from build123d import *

# Parameters (mm, degrees)
SKETCH_1_R      = 3.4
SKETCH_1_R_2    = 3
EXTRUDE_1_DEPTH = 100


with BuildPart() as part:
    # 草图1 → 凸台-拉伸1 (new body)
    with BuildSketch(Plane.XY):
        with BuildLine():
            Line((-5.280003001, 19.242987377), (-15.680003001, 19.242987377))
            ThreePointArc((-15.680003001, 19.242987377), (-18.861983517, 17.924967893), (-20.180003001, 14.742987377))
            Line((-20.180003001, 14.742987377), (-20.180003001, 4.342987377))
            Line((-20.180003001, 4.342987377), (-19.480003001, 4.342987377))
            ThreePointArc((-19.480003001, 4.342987377), (-19.267870967, 4.255119412), (-19.180003001, 4.042987377))
            Line((-19.180003001, 4.042987377), (-19.180003001, 3.342987377))
            Line((-19.180003001, 3.342987377), (-15.980003001, 3.342987377))
            ThreePointArc((-15.980003001, 3.342987377), (-15.767870967, 3.430855343), (-15.680003001, 3.642987377))
            Line((-15.680003001, 3.642987377), (-15.680003001, 6.042987377))
            ThreePointArc((-15.680003001, 6.042987377), (-15.767870967, 6.255119412), (-15.980003001, 6.342987377))
            Line((-15.980003001, 6.342987377), (-16.480003001, 6.342987377))
            ThreePointArc((-16.480003001, 6.342987377), (-17.187109783, 6.635880596), (-17.480003001, 7.342987377))
            Line((-17.480003001, 7.342987377), (-17.480003001, 8.492987377))
            ThreePointArc((-17.480003001, 8.492987377), (-17.187109783, 9.200094158), (-16.480003001, 9.492987377))
            Line((-16.480003001, 9.492987377), (-12.933161007, 9.492987377))
            Line((-12.933161007, 9.492987377), (-8.515789439, 5.07561581))
            ThreePointArc((-8.515789439, 5.07561581), (-8.082243936, 4.426769112), (-7.930003001, 3.661402247))
            Line((-7.930003001, 3.661402247), (-7.930003001, -5.175427493))
            ThreePointArc((-7.930003001, -5.175427493), (-8.082243936, -5.940794357), (-8.515789439, -6.589641055))
            Line((-8.515789439, -6.589641055), (-12.933161007, -11.007012623))
            Line((-12.933161007, -11.007012623), (-16.480003001, -11.007012623))
            ThreePointArc((-16.480003001, -11.007012623), (-17.187109783, -10.714119404), (-17.480003001, -10.007012623))
            Line((-17.480003001, -10.007012623), (-17.480003001, -8.857012623))
            ThreePointArc((-17.480003001, -8.857012623), (-17.187109783, -8.149905842), (-16.480003001, -7.857012623))
            Line((-16.480003001, -7.857012623), (-15.980003001, -7.857012623))
            ThreePointArc((-15.980003001, -7.857012623), (-15.767870967, -7.769144657), (-15.680003001, -7.557012623))
            Line((-15.680003001, -7.557012623), (-15.680003001, -5.157012623))
            ThreePointArc((-15.680003001, -5.157012623), (-15.767870967, -4.944880588), (-15.980003001, -4.857012623))
            Line((-15.980003001, -4.857012623), (-19.180003001, -4.857012623))
            Line((-19.180003001, -4.857012623), (-19.180003001, -5.557012623))
            ThreePointArc((-19.180003001, -5.557012623), (-19.267870967, -5.769144657), (-19.480003001, -5.857012623))
            Line((-19.480003001, -5.857012623), (-20.180003001, -5.857012623))
            Line((-20.180003001, -5.857012623), (-20.180003001, -16.257012623))
            ThreePointArc((-20.180003001, -16.257012623), (-18.861983517, -19.438993138), (-15.680003001, -20.757012623))
            Line((-15.680003001, -20.757012623), (-5.280003001, -20.757012623))
            Line((-5.280003001, -20.757012623), (-5.280003001, -20.057012623))
            ThreePointArc((-5.280003001, -20.057012623), (-5.192135036, -19.844880588), (-4.980003001, -19.757012623))
            Line((-4.980003001, -19.757012623), (-4.280003001, -19.757012623))
            Line((-4.280003001, -19.757012623), (-4.280003001, -16.557012623))
            ThreePointArc((-4.280003001, -16.557012623), (-4.367870967, -16.344880588), (-4.580003001, -16.257012623))
            Line((-4.580003001, -16.257012623), (-6.980003001, -16.257012623))
            ThreePointArc((-6.980003001, -16.257012623), (-7.192135036, -16.344880588), (-7.280003001, -16.557012623))
            Line((-7.280003001, -16.557012623), (-7.280003001, -17.057012623))
            ThreePointArc((-7.280003001, -17.057012623), (-7.57289622, -17.764119404), (-8.280003001, -18.057012623))
            Line((-8.280003001, -18.057012623), (-9.430003001, -18.057012623))
            ThreePointArc((-9.430003001, -18.057012623), (-10.137109783, -17.764119404), (-10.430003001, -17.057012623))
            Line((-10.430003001, -17.057012623), (-10.430003001, -13.510170628))
            Line((-10.430003001, -13.510170628), (-6.012631434, -9.09279906))
            ThreePointArc((-6.012631434, -9.09279906), (-5.363784736, -8.659253558), (-4.598417871, -8.507012623))
            Line((-4.598417871, -8.507012623), (4.238411868, -8.507012623))
            ThreePointArc((4.238411868, -8.507012623), (5.003778733, -8.659253558), (5.652625431, -9.09279906))
            Line((5.652625431, -9.09279906), (10.069996999, -13.510170628))
            Line((10.069996999, -13.510170628), (10.069996999, -17.057012623))
            ThreePointArc((10.069996999, -17.057012623), (9.77710378, -17.764119404), (9.069996999, -18.057012623))
            Line((9.069996999, -18.057012623), (7.919996999, -18.057012623))
            ThreePointArc((7.919996999, -18.057012623), (7.212890217, -17.764119404), (6.919996999, -17.057012623))
            Line((6.919996999, -17.057012623), (6.919996999, -16.557012623))
            ThreePointArc((6.919996999, -16.557012623), (6.832129033, -16.344880588), (6.619996999, -16.257012623))
            Line((6.619996999, -16.257012623), (4.219996999, -16.257012623))
            ThreePointArc((4.219996999, -16.257012623), (4.007864964, -16.344880588), (3.919996999, -16.557012623))
            Line((3.919996999, -16.557012623), (3.919996999, -19.757012623))
            Line((3.919996999, -19.757012623), (4.619996999, -19.757012623))
            ThreePointArc((4.619996999, -19.757012623), (4.832129033, -19.844880588), (4.919996999, -20.057012623))
            Line((4.919996999, -20.057012623), (4.919996999, -20.757012623))
            Line((4.919996999, -20.757012623), (15.319996999, -20.757012623))
            ThreePointArc((15.319996999, -20.757012623), (18.501977514, -19.438993138), (19.819996999, -16.257012623))
            Line((19.819996999, -16.257012623), (19.819996999, -5.857012623))
            Line((19.819996999, -5.857012623), (19.119996999, -5.857012623))
            ThreePointArc((19.119996999, -5.857012623), (18.907864964, -5.769144657), (18.819996999, -5.557012623))
            Line((18.819996999, -5.557012623), (18.819996999, -4.857012623))
            Line((18.819996999, -4.857012623), (15.619996999, -4.857012623))
            ThreePointArc((15.619996999, -4.857012623), (15.407864964, -4.944880588), (15.319996999, -5.157012623))
            Line((15.319996999, -5.157012623), (15.319996999, -7.557012623))
            ThreePointArc((15.319996999, -7.557012623), (15.407864964, -7.769144657), (15.619996999, -7.857012623))
            Line((15.619996999, -7.857012623), (16.119996999, -7.857012623))
            ThreePointArc((16.119996999, -7.857012623), (16.82710378, -8.149905842), (17.119996999, -8.857012623))
            Line((17.119996999, -8.857012623), (17.119996999, -10.007012623))
            ThreePointArc((17.119996999, -10.007012623), (16.82710378, -10.714119404), (16.119996999, -11.007012623))
            Line((16.119996999, -11.007012623), (12.573155004, -11.007012623))
            Line((12.573155004, -11.007012623), (8.155783436, -6.589641055))
            ThreePointArc((8.155783436, -6.589641055), (7.722237934, -5.940794357), (7.569996999, -5.175427493))
            Line((7.569996999, -5.175427493), (7.569996999, 3.661402247))
            ThreePointArc((7.569996999, 3.661402247), (7.722237934, 4.426769112), (8.155783436, 5.07561581))
            Line((8.155783436, 5.07561581), (12.573155004, 9.492987377))
            Line((12.573155004, 9.492987377), (16.119996999, 9.492987377))
            ThreePointArc((16.119996999, 9.492987377), (16.82710378, 9.200094158), (17.119996999, 8.492987377))
            Line((17.119996999, 8.492987377), (17.119996999, 7.342987377))
            ThreePointArc((17.119996999, 7.342987377), (16.82710378, 6.635880596), (16.119996999, 6.342987377))
            Line((16.119996999, 6.342987377), (15.619996999, 6.342987377))
            ThreePointArc((15.619996999, 6.342987377), (15.407864964, 6.255119412), (15.319996999, 6.042987377))
            Line((15.319996999, 6.042987377), (15.319996999, 3.642987377))
            ThreePointArc((15.319996999, 3.642987377), (15.407864964, 3.430855343), (15.619996999, 3.342987377))
            Line((15.619996999, 3.342987377), (18.819996999, 3.342987377))
            Line((18.819996999, 3.342987377), (18.819996999, 4.042987377))
            ThreePointArc((18.819996999, 4.042987377), (18.907864964, 4.255119412), (19.119996999, 4.342987377))
            Line((19.119996999, 4.342987377), (19.819996999, 4.342987377))
            Line((19.819996999, 4.342987377), (19.819996999, 14.742987377))
            ThreePointArc((19.819996999, 14.742987377), (18.501977514, 17.924967893), (15.319996999, 19.242987377))
            Line((15.319996999, 19.242987377), (4.919996999, 19.242987377))
            Line((4.919996999, 19.242987377), (4.919996999, 18.542987377))
            ThreePointArc((4.919996999, 18.542987377), (4.832129033, 18.330855343), (4.619996999, 18.242987377))
            Line((4.619996999, 18.242987377), (3.919996999, 18.242987377))
            Line((3.919996999, 18.242987377), (3.919996999, 15.042987377))
            ThreePointArc((3.919996999, 15.042987377), (4.007864964, 14.830855343), (4.219996999, 14.742987377))
            Line((4.219996999, 14.742987377), (6.619996999, 14.742987377))
            ThreePointArc((6.619996999, 14.742987377), (6.832129033, 14.830855343), (6.919996999, 15.042987377))
            Line((6.919996999, 15.042987377), (6.919996999, 15.542987377))
            ThreePointArc((6.919996999, 15.542987377), (7.212890217, 16.250094158), (7.919996999, 16.542987377))
            Line((7.919996999, 16.542987377), (9.069996999, 16.542987377))
            ThreePointArc((9.069996999, 16.542987377), (9.77710378, 16.250094158), (10.069996999, 15.542987377))
            Line((10.069996999, 15.542987377), (10.069996999, 11.996145383))
            Line((10.069996999, 11.996145383), (5.652625431, 7.578773815))
            ThreePointArc((5.652625431, 7.578773815), (5.003778733, 7.145228312), (4.238411868, 6.992987377))
            Line((4.238411868, 6.992987377), (-4.598417871, 6.992987377))
            ThreePointArc((-4.598417871, 6.992987377), (-5.363784736, 7.145228312), (-6.012631434, 7.578773815))
            Line((-6.012631434, 7.578773815), (-10.430003001, 11.996145383))
            Line((-10.430003001, 11.996145383), (-10.430003001, 15.542987377))
            ThreePointArc((-10.430003001, 15.542987377), (-10.137109783, 16.250094158), (-9.430003001, 16.542987377))
            Line((-9.430003001, 16.542987377), (-8.280003001, 16.542987377))
            ThreePointArc((-8.280003001, 16.542987377), (-7.57289622, 16.250094158), (-7.280003001, 15.542987377))
            Line((-7.280003001, 15.542987377), (-7.280003001, 15.042987377))
            ThreePointArc((-7.280003001, 15.042987377), (-7.192135036, 14.830855343), (-6.980003001, 14.742987377))
            Line((-6.980003001, 14.742987377), (-4.580003001, 14.742987377))
            ThreePointArc((-4.580003001, 14.742987377), (-4.367870967, 14.830855343), (-4.280003001, 15.042987377))
            Line((-4.280003001, 15.042987377), (-4.280003001, 18.242987377))
            Line((-4.280003001, 18.242987377), (-4.980003001, 18.242987377))
            ThreePointArc((-4.980003001, 18.242987377), (-5.192135036, 18.330855343), (-5.280003001, 18.542987377))
            Line((-5.280003001, 18.542987377), (-5.280003001, 19.242987377))
        make_face()
        with Locations((-0.180003001, -0.757012623)):
            Circle(SKETCH_1_R, mode=Mode.SUBTRACT)
        with Locations((-15.305003001, 14.367987377)):
            Circle(SKETCH_1_R_2, mode=Mode.SUBTRACT)
        with Locations((14.944996999, 14.367987377)):
            Circle(SKETCH_1_R_2, mode=Mode.SUBTRACT)
        with Locations((-15.305003001, -15.882012623)):
            Circle(SKETCH_1_R_2, mode=Mode.SUBTRACT)
        with Locations((14.944996999, -15.882012623)):
            Circle(SKETCH_1_R_2, mode=Mode.SUBTRACT)
    extrude(amount=EXTRUDE_1_DEPTH)


solid = part.part
Geometry: final body of the model. Coordinates: model frame, mm. A direction names the side the tool comes from. Coordinates: 2 decimals unless noted, no trailing zeros. Write each loop counter-clockwise with the first axis right and the second up, starting at its lowest first coordinate (ties: lowest second). Pieces come first, ordered by that corner, then holes. Notation, with made-up numbers: (67, 1) - (92, 1) arc R5 ccw to (92, 7) - close; hole circle Ø2 at (-16, 30.5). An arc over 180 degrees is marked (long way). Return JSON: item names as keys, results as strings.
Item 1: Pin query (flat end, axial travel): pin 1 Ø1.6 at (x, z) = (18, 51.5) entering from -Y; pin 2 Ø2.5 at (y, z) = (16.5, 26.5) entering from +X; pin 3 Ø0.6 at (y, z) = (-17, 54) entering from -X; pin 4 Ø1 at (x, y) = (14.5, -9.5) entering from +Z. Return the tip coordinate at first contact, or that it passes through.
Completed:
{"pin 1": "stops at y = -20.35", "pin 2": "stops at x = 19.79", "pin 3": "stops at x = -20.16", "pin 4": "passes through"}
Item 2: Section query C-C (z = 36). Count the separate pieces of the cut face and the enclosed holes in it, and give its area (3 significant figures).
Completed:
{"separate pieces": "1", "enclosed holes": "5", "area": "701 mm2"}
Item 3: Section query A-A (x = -14). Output: boundary loops of the cut face in (y, z).
Completed:
{"outline": "(-20.76, 0) - (-18.58, 0) - (-18.58, 100) - (-20.76, 100) - close; (-13.18, 0) - (-11.01, 0) - (-11.01, 100) - (-13.18, 100) - close; (9.49, 0) - (11.67, 0) - (11.67, 100) - (9.49, 100) - close; (17.07, 0) - (19.24, 0) - (19.24, 100) - (17.07, 100) - close"}
Item 4: Reachability of faces 4 (the face through (15.32, -6, 49)), 5 (the face through (-4.28, -18, 49)), 6 (the face through (-4.28, 17, 49)) from +Z, -Z, +X, -X, +Y, -Y: full face, straight path, thin tool, end or side. Return the list, or none.
Completed:
{"face 4": "+Z, -Z", "face 5": "+Z, -Z, -Y", "face 6": "+Z, -Z, +Y"}
Item 5: Line query: L1, parallel to X at y = -17.5, z = 45; L2, parallel to X at y = -5.5, z = 64.5; L3, parallel to X at y = 11, z = 92.5. Output: solid intervals per line, ascending.
Completed:
{"L1": "x = -20 to -17.83, -12.78 to -10.33, -7.38 to -4.28, 3.92 to 7.02, 9.97 to 12.42, 17.47 to 19.64", "L2": "x = -19.18 to -15.68, -7.96 to 7.6, 15.32 to 18.82", "L3": "x = -20.18 to -9.43, 9.07 to 19.82"}
Item 6: Pull-direction query (Y, two-part tool) for faces 1 (the face through (10, -20.757, 49)), 2 (the face through (18.537, 17.89, 49.3)), 3 (the face through (7.57, -1, 49)); classes: +Y half, -Y half, draft (parallel to the pull), parting line (faces both ways), or undercut.
Completed:
{"face 1": "-Y half", "face 2": "+Y half", "face 3": "undercut"}
Item 7: Section query B-B (x = -1). Output: boundary loops of the cut face in (y, z).
Completed:
{"outline": "(-8.51, 0) - (-4.06, 0) - (-4.06, 100) - (-8.51, 100) - close; (2.54, 0) - (6.99, 0) - (6.99, 100) - (2.54, 100) - close"}
